Check sheet for the modelled part. Datum: model origin and axes. Units: mm. Face numbers are marked on the shaded views. Round coordinates to 2 decimals unless told otherwise and drop trailing zeros. Order: outer loops, then holes, each group sorted by start corner. A loop starts at its lowest first (then second) coordinate and runs counter-clockwise, first axis right, second up. Notation, with made-up numbers: M 74,0 L 126,0 A21 ccw 126,32 Z; hole C 47.25,-8.5 d9. An arc over 180 degrees is marked long. One line per item, written item: value. Start each with the question number.
(1) Cross-section at C-C, the plane x = 46. Enter the section's corners in (y, z), and give its area (3 significant figures).
(2) Cross-section at B-B, the plane y = 13. Enter the section's corners in (x, z), and give its area (3 significant figures).
(3) Release check for a two-part mould opening along X. For the marked faces 1, 2 and 3 record: released by +X, released by -X, zero draft, split by the parting line, or undercut.
(4) Thickness scan on L1, parallel to Y at x = 30, z = 14; L2, parallel to Y at x = 30, z = 2.9; L3, parallel to X at y = 12.5, z = 1. Record the ranges inside material, lowest first.
(5) Cross-section at A-A, the plane z = 10.1. Enter the section's corners in (x, y).
(6) Cross-section at D-D, the plane z = 16.5. Enter the section's corners in (x, y), and give its area (3 significant figures).
(7) Depth check by flat-ended pin: pin 1 Ø14.5 at (x, y) = (30, 13) entering from +Z. Enter the tip coordinate at first touch or a pass-through.
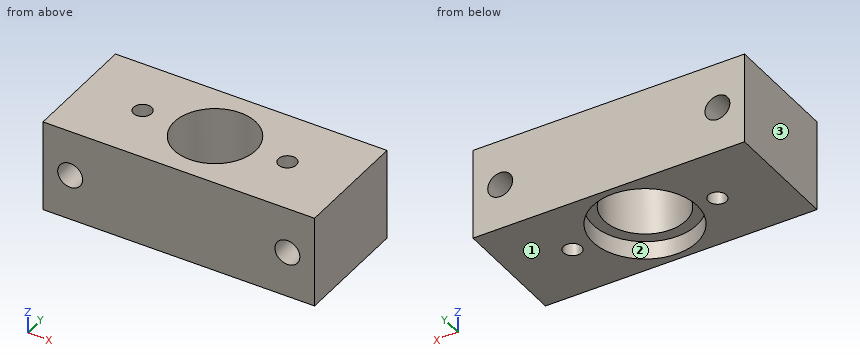
from build123d import *

# Parameters (mm, degrees)
SKETCH1_W                      = 60
SKETCH1_H                      = 26
BOSS_EXTRUDE1_DEPTH            = 20.2
SKETCH2_R                      = 9
SKETCH2_R_2                    = 2
CUT_EXTRUDE1_DEPTH             = 69.440046756
SKETCH3_R                      = 11.5
CUT_EXTRUDE2_DEPTH             = 4
F_5_5_5_5_DIAMETER_HOLE1_D     = 5.5
F_5_5_5_5_DIAMETER_HOLE1_DEPTH = 30
F_5_5_5_5_DIAMETER_HOLE1_TIP   = 1.652366702


with BuildPart() as part:
    # Sketch1 → Boss-Extrude1 (new body)
    with BuildSketch(Plane.XY):
        with Locations((30, 13)):
            Rectangle(SKETCH1_W, SKETCH1_H)
    extrude(amount=BOSS_EXTRUDE1_DEPTH)

    # Sketch2 → Cut-Extrude1 (cut, through all)
    with BuildSketch(Plane.XY.offset(20.2)):
        with Locations((30, 13)):
            Circle(SKETCH2_R)
        with Locations((14, 13)):
            Circle(SKETCH2_R_2)
        with Locations((46, 13)):
            Circle(SKETCH2_R_2)
    extrude(amount=-CUT_EXTRUDE1_DEPTH, mode=Mode.SUBTRACT)

    # Sketch3 → Cut-Extrude2 (cut)
    with BuildSketch(Plane(origin=(0, 0, 0), x_dir=(-1, 0, 0), z_dir=(0, 0, -1))):
        with Locations((-30, 13)):
            Circle(SKETCH3_R)
    extrude(amount=-CUT_EXTRUDE2_DEPTH, mode=Mode.SUBTRACT)

    # Ø5.5 (5.5) Diameter Hole1
    with Locations(Plane(origin=(0, 26, 0), x_dir=(-1, 0, 0), z_dir=(0, 1, 0))):
        with Locations((-6, 10.1), (-54, 10.1)):
            Hole(F_5_5_5_5_DIAMETER_HOLE1_D / 2, depth=F_5_5_5_5_DIAMETER_HOLE1_DEPTH)
            with Locations((0, 0, -(F_5_5_5_5_DIAMETER_HOLE1_DEPTH + F_5_5_5_5_DIAMETER_HOLE1_TIP / 2))):  # 118° drill point
                Cone(0, F_5_5_5_5_DIAMETER_HOLE1_D / 2, F_5_5_5_5_DIAMETER_HOLE1_TIP, mode=Mode.SUBTRACT)


solid = part.part
Values found:
1. outline: M 0,0 L 11,0 L 11,20.2 L 0,20.2 Z; M 15,0 L 26,0 L 26,20.2 L 15,20.2 Z
1. area: 444 mm^2
2. outline: M 0,0 L 12,0 L 12,20.2 L 0,20.2 Z; M 16,0 L 18.5,0 L 18.5,4 L 21,4 L 21,20.2 L 16,20.2 Z; M 39,4 L 41.5,4 L 41.5,0 L 44,0 L 44,20.2 L 39,20.2 Z; M 48,0 L 60,0 L 60,20.2 L 48,20.2 Z; hole C 6,10.1 d5.5; hole C 54,10.1 d5.5
2. area: 619 mm^2
3. face 1: zero draft
3. face 2: undercut
3. face 3: released by -X
4. L1: 0 to 4, 22 to 26
4. L2: 0 to 1.5, 24.5 to 26
4. L3: 0 to 12.06, 15.94 to 18.51, 41.49 to 44.06, 47.94 to 60
5. outline: M 0,0 L 3.25,0 L 3.25,26 L 0,26 Z; M 8.75,0 L 51.25,0 L 51.25,26 L 8.75,26 Z; M 56.75,0 L 60,0 L 60,26 L 56.75,26 Z; hole C 14,13 d4; hole C 30,13 d18; hole C 46,13 d4
6. outline: M 0,0 L 60,0 L 60,26 L 0,26 Z; hole C 14,13 d4; hole C 30,13 d18; hole C 46,13 d4
6. area: 1,280 mm^2
7. pin 1: through
